```python
from build123d import *

# Parameters (mm, degrees)
SKETCH1_W           = 43.412860342
SKETCH1_H           = 140
BOSS_EXTRUDE1_DEPTH = 50
SKETCH2_R           = 5
CUT_EXTRUDE1_DEPTH  = 50
SKETCH3_W           = 30
SKETCH3_H           = 30
CUT_EXTRUDE2_DEPTH  = 50
SKETCH5_R           = 15
CUT_EXTRUDE3_DEPTH  = 50


with BuildPart() as part:
    # Sketch1 → Boss-Extrude1 (new body)
    with BuildSketch(Plane.XY):
        with Locations((230.409564966, -45)):
            Rectangle(SKETCH1_W, SKETCH1_H)
        with Locations((230.409564966, -185)):
            Rectangle(SKETCH1_W, SKETCH1_H)
    extrude(amount=BOSS_EXTRUDE1_DEPTH)

    # Sketch2 → Cut-Extrude1 (cut)
    with BuildSketch(Plane.XY.offset(50)):
        with Locations((230, 0)):
            Circle(SKETCH2_R)
        with Locations((230, -230)):
            Circle(SKETCH2_R)
    extrude(amount=-CUT_EXTRUDE1_DEPTH, mode=Mode.SUBTRACT)

    # Sketch3 → Cut-Extrude2 (cut)
    with BuildSketch(Plane(origin=(252.115995137, 0, 0), x_dir=(0, 0, -1), z_dir=(1, 0, 0))):
        with Locations((-25, 0)):
            Rectangle(SKETCH3_W, SKETCH3_H)
        with Locations((-25, -230)):
            Rectangle(SKETCH3_W, SKETCH3_H)
    extrude(amount=-CUT_EXTRUDE2_DEPTH, mode=Mode.SUBTRACT)

    # Sketch5 → Cut-Extrude3 (cut)
    with BuildSketch(Plane(origin=(252.115995137, 0, 0), x_dir=(0, 0, -1), z_dir=(1, 0, 0))):
        with Locations(Location((-25, -115, 0), (0, 0, 90))):
            Circle(SKETCH5_R)
    extrude(amount=-CUT_EXTRUDE3_DEPTH, mode=Mode.SUBTRACT)


solid = part.part
```
For this review, take the finished solid that the model builds, in its own axes (mm). A direction names the side the tool comes from. Give positions to 0.01 mm unless a question says otherwise; leave off trailing zeros. Loops run counter-clockwise (first coordinate to the right, second up) from the corner with the lowest first, then second, coordinate; pieces in that order, holes last. Notation, with made-up numbers: M -37.5,23 L -17.5,23 A13 cw -17.5,44 Z; hole C 74.5,-11 d8. An arc over 180 degrees is marked long. One line per item, written item: value. Start each with the question number.
Q1. Add section B-B (x = 230). Count the separate pieces of the cut face and the enclosed holes in it, and give its area (3 significant figures).
Q2. Add section D-D (z = 25). Give the boundary of the cut face in (x, y).
Q3. Draft analysis for pull direction X (two halves, no side actions). For faces 3 (the face through (252.116, -117, 8)), 4 (the face through (234.77, 1.5, 5.07)), 5 (the face through (230, -113, 50)), state which applies: released by +X, released by -X, zero draft, split by the parting line, or undercut.
Q4. Machinability: for faces 1 (the face through (234.77, -228.5, 5.07)), 2 (the face through (231, -15, 25)), which of the approach directions +Z, -Z, +X, -X, +Y, -Y give a long, thin tool a straight path to every point of the face, cutting with its end or side? Answer none if there is none.
Q5. For L1, parallel to Y at x = 235, z = 26; L2, parallel to Y at x = 230, z = 3; L3, parallel to Z at x = 240, y = -115, list the stretches that pass through material, from the lowest coordinate up.
Q6. Add section A-A (y = 0). Give the boundary of the cut face in (x, z).
Q7. Add section C-C (y = -115). Give the boundary of the cut face in (x, z).
Q8. Clearance check with a flat-ended pin moving along its axis: pin 1 Ø6 at (x, y) = (221.5, -98) entering from -Z. State where the tip first meets the part, or that it passes through.
Reply:
1. separate pieces: 3
1. enclosed holes: 1
1. area: 11,100 mm²
2. outline: M 208.7,-255 L 252.12,-255 L 252.12,-245 L 208.7,-245 Z; M 208.7,-215 L 252.12,-215 L 252.12,-130 L 208.7,-130 Z; M 208.7,-100 L 252.12,-100 L 252.12,-15 L 208.7,-15 Z; M 208.7,15 L 252.12,15 L 252.12,25 L 208.7,25 Z
3. face 3: released by +X
3. face 4: undercut
3. face 5: zero draft
4. face 1: +Z, -Z
4. face 2: +X, -X
5. L1: -255 to -245, -215 to -129.97, -100.03 to -15, 15 to 25
5. L2: -255 to -235, -225 to -5, 5 to 25
5. L3: 0 to 10, 40 to 50
6. outline: M 208.7,0 L 225,0 L 225,10 L 208.7,10 Z; M 208.7,40 L 225,40 L 225,50 L 208.7,50 Z; M 235,0 L 252.12,0 L 252.12,10 L 235,10 Z; M 235,40 L 252.12,40 L 252.12,50 L 235,50 Z
7. outline: M 208.7,0 L 252.12,0 L 252.12,10 L 208.7,10 Z; M 208.7,40 L 252.12,40 L 252.12,50 L 208.7,50 Z
8. pin 1: z = 0
